```python
from build123d import *

# Parameters (mm, degrees)
F0_W      = 100
F0_H      = 15
F0_W_2    = 63
F0_H_2    = 3
F1_DEPTH  = 4
F2_W      = 69
F2_H      = 15
F3_DEPTH  = 2
F4_R      = 2.5
F5_DEPTH  = 25
F6_R      = 2.5
F7_DEPTH  = 25
F8_W      = 9
F8_H      = 3
F9_DEPTH  = 2
F10_R     = 1.5
F11_DEPTH = 25


with BuildPart() as f1:
    # F0 (on Front) → F1 (new body)
    with BuildSketch(Plane.XZ):
        Rectangle(F0_W, F0_H)
        with Locations((0, -3)):
            Rectangle(F0_W_2, F0_H_2, mode=Mode.SUBTRACT)
        with Locations((0, 3)):
            Rectangle(F0_W_2, F0_H_2, mode=Mode.SUBTRACT)
    extrude(amount=F1_DEPTH)

    # F2 (on face) → F3 (cut)
    with BuildSketch(Plane(origin=(0, 0, 0), x_dir=(-1, 0, 0), z_dir=(0, 1, 0))):
        Rectangle(F2_W, F2_H)
    extrude(amount=-F3_DEPTH, mode=Mode.SUBTRACT)

    # F4 (on face) → F5 (cut)
    with BuildSketch(Plane(origin=(0, 0, 0), x_dir=(-1, 0, 0), z_dir=(0, 1, 0))):
        with Locations((-42.25, 0)):
            Circle(F4_R)
    extrude(amount=-F5_DEPTH, mode=Mode.SUBTRACT)

    # F6 (on face) → F7 (cut)
    with BuildSketch(Plane(origin=(0, 0, 0), x_dir=(-1, 0, 0), z_dir=(0, 1, 0))):
        with Locations((42.25, 0)):
            Circle(F6_R)
    extrude(amount=-F7_DEPTH, mode=Mode.SUBTRACT)

    # F8 (on face) → F9 (join)
    with BuildSketch(Plane.XZ.offset(4)):
        with Locations((27, 3)):
            Rectangle(F8_W, F8_H)
    extrude(amount=-F9_DEPTH)

    # F10 (on face) → F11 (cut)
    with BuildSketch(Plane.XZ.offset(4)):
        with Locations((27, 3)):
            Circle(F10_R)
    extrude(amount=-F11_DEPTH, mode=Mode.SUBTRACT)


solid = f1.part
```
Model file for the job. Use its own axes, mm. A direction names the side the tool comes from. Give positions to 0.01 mm unless a question says otherwise; leave off trailing zeros. Write each loop counter-clockwise with the first axis right and the second up, starting at its lowest first coordinate (ties: lowest second). Pieces come first, ordered by that corner, then holes. Notation, with made-up numbers: (23.25, 23.5) -> (76.25, 23.5) arc R18 cw to (76.25, 37.5) -> close; hole circle Ø1 at (31, -16). An arc over 180 degrees is marked (long way). Use CSV: the item, a comma, the result in double quotes. Start each with the question number.
1) Two-plate mould, pull along X, no slides. Class faces 1 (the flat face through (-31.5, -3, 3)), 2 (the flat face through (-1, -4, 0)), 3 (the flat face through (50, -2, 0)): released by +X, released by -X, zero draft, split by the parting line, or undercut.
2) Cut at C-C on z = 0. List the corners of the cut face in (x, y), plus the area to 3 significant figures.
3) Tool access for faces 4 (the flat face through (-34.5, -1, 0)), 5 (the flat face through (-44, 0, 2)), 6 (the flat face through (-5, -3, 1.5)): list every direction of +Z, -Z, +X, -X, +Y, -Y with a clear straight run to the whole face (end or side of a thin tool).
4) Drill centre lines: L1, parallel to Z at x = -12, y = -2.1; L2, parallel to X at y = -1.85, z = 4.25; L3, parallel to Z at x = 42.25, y = -1.4. Where is each one in solid material? Low to high.
5) Cut at B-B on y = -2.7. List the corners of the cut face in (x, z), plus the area to 3 significant figures.
6) Cut at A-A on x = 27. List the corners of the cut face in (y, z), plus the area to 3 significant figures.
7) Cut at D-D on x = -42.25. List the corners of the cut face in (y, z).
8) Pin check, flat tip, straight feed: P1, Ø7.5, axis at x = -5.5, z = 1.5, coming from the +Y side. Stop position of the tip, or through.
Final values:
1,face 1,"undercut"
1,face 2,"zero draft"
1,face 3,"released by +X"
2,outline,"(-50, -4) -> (-44.75, -4) -> (-44.75, 0) -> (-50, 0) -> close; (-39.75, -4) -> (39.75, -4) -> (39.75, 0) -> (34.5, 0) -> (34.5, -2) -> (-34.5, -2) -> (-34.5, 0) -> (-39.75, 0) -> close; (44.75, -4) -> (50, -4) -> (50, 0) -> (44.75, 0) -> close"
2,area,"222 mm2"
3,face 4,"+Z, -Z, +Y"
3,face 5,"+Z, -Z, +X, -X, +Y"
3,face 6,"+Y, -Y"
4,L1,"z = -7.5 to -4.5, -1.5 to 1.5, 4.5 to 7.5"
4,L2,"x = -50 to -34.5, 34.5 to 50"
4,L3,"z = -7.5 to -2.5, 2.5 to 7.5"
5,outline,"(-50, -7.5) -> (50, -7.5) -> (50, 7.5) -> (-50, 7.5) -> close; hole circle Ø5 at (-42.25, 0); hole (-31.5, -4.5) -> (31.5, -4.5) -> (31.5, -1.5) -> (-31.5, -1.5) -> close; hole (-31.5, 1.5) -> (22.5, 1.5) -> (22.5, 4.5) -> (-31.5, 4.5) -> close; hole circle Ø3 at (27, 3); hole circle Ø5 at (42.25, 0)"
5,area,"1,100 mm2"
6,outline,"(-4, -7.5) -> (-2, -7.5) -> (-2, -4.5) -> (-4, -4.5) -> close; (-4, -1.5) -> (-2, -1.5) -> (-2, 1.5) -> (-4, 1.5) -> close; (-4, 4.5) -> (-2, 4.5) -> (-2, 7.5) -> (-4, 7.5) -> close"
6,area,"18.0 mm2"
7,outline,"(-4, -7.5) -> (0, -7.5) -> (0, -2.5) -> (-4, -2.5) -> close; (-4, 2.5) -> (0, 2.5) -> (0, 7.5) -> (-4, 7.5) -> close"
8,P1,"stops at y = -2"
